```python
from build123d import *

# Parameters (mm, degrees)
F0_W     = 25.530833751
F0_H     = 31.9637935609
F1_DEPTH = 25.4
F2_W     = 12.830833751
F2_H     = 6.35
F3_DEPTH = 25.401
F4_DEPTH = 12.7
F5_W     = 12.7
F5_H     = 6.35
F6_DEPTH = 25.531833751


with BuildPart() as f1:
    # F0 (on Front) → F1 (new body)
    with BuildSketch(Plane.XZ):
        with Locations((-45.3322995454, 40.3065467253)):
            Rectangle(F0_W, F0_H)
    extrude(amount=F1_DEPTH)

    # F2 (on face) → F3 (cut, through all)
    with BuildSketch(Plane(origin=(0, 0, 0), x_dir=(-1, 0, 0), z_dir=(0, 1, 0))):
        with Locations((45.3322995454, 53.1134435058)):
            Rectangle(F2_W, F2_H)
    extrude(amount=-F3_DEPTH, mode=Mode.SUBTRACT)

    # F4 (add): a face of the model
    f4_faces = [f1.faces().sort_by_distance(p)[0] for p in [
        (-45.3322995454, -25.4, 38.8860849),
    ]]
    extrude(f4_faces, amount=F4_DEPTH)

    # F5 (on face) → F6 (cut, through all)
    with BuildSketch(Plane.YZ.offset(-32.5668826699)):
        with Locations((-19.05, 27.4996499449)):
            Rectangle(F5_W, F5_H)
    extrude(amount=-F6_DEPTH, mode=Mode.SUBTRACT)


solid = f1.part
```
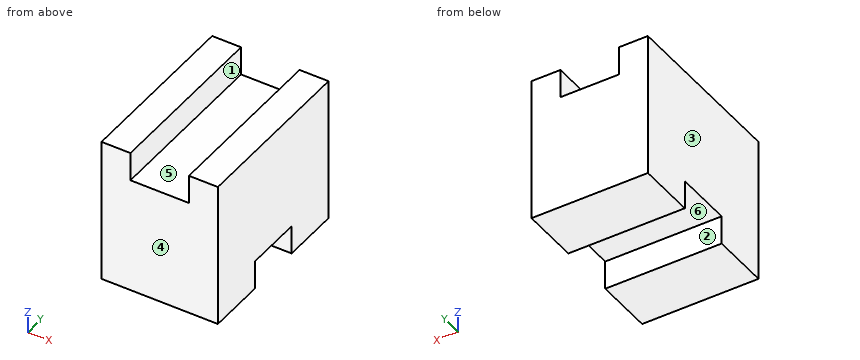
Part model, mm, in its own coordinate system. Face numbers are marked on the shaded views. A direction names the side the tool comes from. Coordinates: 2 decimals unless noted, no trailing zeros. Order: outer loops, then holes, each group sorted by start corner. A loop starts at its lowest first (then second) coordinate and runs counter-clockwise, first axis right, second up. Notation, with made-up numbers: (-37, -28.75) - (11, -28.75) arc R25 cw to (11, 2.25) - close; hole circle Ø9 at (-30, 48). An arc over 180 degrees is marked (long way). Return JSON: item names as keys, results as strings. Group by question number.
Item 1: Cut at C-C (x = -56.25). List the corners of the cut face in (y, z), plus the area to 3 significant figures.
Item 2: Which spindle directions (+Z, -Z, +X, -X, +Y, -Y) get a long thin tool onto all of the face, cutting with end or side? Do the marked faces 1, 2 and 3. Say none if no direction does.
Item 3: Pin check, flat tips, straight feed: pin 1 (6.5 mm diameter, centred on x = -44, y = -19, fed in from -Z); pin 2 (10.5 mm diameter, centred on x = -45.5, y = -25.5, fed in from +Z). Stop position of each tip, or through.
Item 4: Cut at A-A (z = 52.5). List the corners of the cut face in (x, y).
Item 5: Cut at B-B (y = -3.5). List the corners of the cut face in (x, z), plus the area to 3 significant figures.
Item 6: Drill centre lines: probe 1 along X at (y, z) = (-21, 53.5); probe 2 along Y at (x, z) = (-53.25, 29); probe 3 along Z at (x, y) = (-45, -9.5). Where is each one in solid material? Low to high. Write a range as from..to.
Item 7: Pull direction Y, two halves, no side cores. Call the marked faces 4, 5 and 6: pulls with the +Y half, pulls with the -Y half, needs draft (parallel to the pull), parting line crosses it, or undercut.
Check values:
{
 "1": {"outline": "(-38.1, 24.32) - (-25.4, 24.32) - (-25.4, 30.67) - (-12.7, 30.67) - (-12.7, 24.32) - (0, 24.32) - (0, 56.29) - (-38.1, 56.29) - close", "area": "1,140 mm2"},
 "2": {"face 1": "+Z, +Y, -Y", "face 2": "-Z, +X, -X", "face 3": "+Z, -Z, -X, +Y, -Y"},
 "3": {"pin 1": "stops at z = 30.67", "pin 2": "stops at z = 49.94"},
 "4": {"outline": "(-58.1, -38.1) - (-51.75, -38.1) - (-51.75, 0) - (-58.1, 0) - close; (-38.92, -38.1) - (-32.57, -38.1) - (-32.57, 0) - (-38.92, 0) - close"},
 "5": {"outline": "(-58.1, 24.32) - (-32.57, 24.32) - (-32.57, 56.29) - (-38.92, 56.29) - (-38.92, 49.94) - (-51.75, 49.94) - (-51.75, 56.29) - (-58.1, 56.29) - close", "area": "735 mm2"},
 "6": {"probe 1": "x = -58.1..-51.75, -38.92..-32.57", "probe 2": "y = -38.1..-25.4, -12.7..0", "probe 3": "z = 24.32..49.94"},
 "7": {"face 4": "pulls with the -Y half", "face 5": "needs draft", "face 6": "undercut"}
}
